The listing builds one solid part. Answer for the finished solid, in the listing's coordinates (mm). A direction names the side the tool comes from. Give positions to 0.01 mm unless a question says otherwise; leave off trailing zeros. Use CSV: the item, a comma, the result in double quotes.
```python
from build123d import *

# Parameters (mm, degrees)
F0_W      = 30
F0_H      = 30
F1_DEPTH  = 15
F3_ANGLE  = 270
F4_R      = 2
F5_R      = 1
F6_DEPTH  = 2
F7_R      = 1
F8_DEPTH  = 2
F10_DEPTH = 2
F11_R     = 1
F12_DEPTH = 2
F13_R     = 1
F14_DEPTH = 2
F15_R     = 1
F16_DEPTH = 2


with BuildPart() as f1:
    # F0 (on Front) → F1 (new body, symmetric)
    with BuildSketch(Plane.XZ):
        Rectangle(F0_W, F0_H)
    extrude(amount=F1_DEPTH, both=True)


with BuildPart() as f1_1:
    # F3: moved
    add(f1.part.rotate(Axis((0, 0.380553, 0), (0, 1, 0)), F3_ANGLE))

    # F4
    f4_edges = [f1_1.edges().sort_by_distance(p)[0] for p in [
        (-15, 0, 15),
        (-15, -15, 0),
        (0, -15, 15),
        (15, -15, 0),
        (15, 0, 15),
        (0, 15, 15),
        (15, 0, -15),
        (0, -15, -15),
        (-15, 0, -15),
        (-15, 15, 0),
        (0, 15, -15),
        (15, 15, 0),
    ]]
    fillet(f4_edges, radius=F4_R)

    # F5 (on face) → F6 (cut)
    with BuildSketch(Plane.XZ.offset(15)):
        Circle(F5_R)
    extrude(amount=-F6_DEPTH, mode=Mode.SUBTRACT)

    # F7 (on face) → F8 (cut)
    with BuildSketch(Plane(origin=(-15, 0, 0), x_dir=(0, -1, 0), z_dir=(-1, 0, 0))):
        with Locations((-10, -10)):
            Circle(F7_R)
        with Locations((10, -10)):
            Circle(F7_R)
        with Locations((10, 10)):
            Circle(F7_R)
        with Locations((-10, 10)):
            Circle(F7_R)
    extrude(amount=-F8_DEPTH, mode=Mode.SUBTRACT)

    # F9 (on face) → F10 (cut)
    with BuildSketch(Plane(origin=(0, 15, 0), x_dir=(-1, 0, 0), z_dir=(0, 1, 0))):
        with BuildLine():
            ThreePointArc((-10, 9), (-9.292893, 9.292893), (-9, 10))
            ThreePointArc((-9, 10), (-10.707107, 10.707107), (-10, 9))
        make_face()
        with BuildLine():
            ThreePointArc((-9, -10), (-9.292893, -9.292893), (-10, -9))
            ThreePointArc((-10, -9), (-10.707107, -10.707107), (-9, -10))
        make_face()
        with BuildLine():
            ThreePointArc((-9, 0), (-9.292893, 0.707107), (-10, 1))
            Line((-10, 1), (-10, -1))
            ThreePointArc((-10, -1), (-9.292893, -0.707107), (-9, 0))
        make_face()
        with BuildLine():
            Line((-10, -1), (-10, 1))
            ThreePointArc((-10, 1), (-11, 0), (-10, -1))
        make_face()
        with BuildLine():
            ThreePointArc((10, -1), (10.707107, -0.707107), (11, 0))
            ThreePointArc((11, 0), (10.707107, 0.707107), (10, 1))
            Line((10, 1), (10, -1))
        make_face()
        with BuildLine():
            ThreePointArc((11, -10), (10.707107, -9.292893), (10, -9))
            ThreePointArc((10, -9), (9.292893, -10.707107), (11, -10))
        make_face()
        with BuildLine():
            ThreePointArc((11, 10), (9.292893, 10.707107), (10, 9))
            ThreePointArc((10, 9), (10.707107, 9.292893), (11, 10))
        make_face()
        with BuildLine():
            Line((10, -1), (10, 1))
            ThreePointArc((10, 1), (9, 0), (10, -1))
        make_face()
    extrude(amount=-F10_DEPTH, mode=Mode.SUBTRACT)

    # F11 (on face) → F12 (cut)
    with BuildSketch(Plane.YZ.offset(15)):
        with Locations((-10, 10)):
            Circle(F11_R)
        with Locations((10, -10)):
            Circle(F11_R)
        Circle(F11_R)
    extrude(amount=-F12_DEPTH, mode=Mode.SUBTRACT)

    # F13 (on face) → F14 (cut)
    with BuildSketch(Plane.XY.offset(15)):
        with Locations((-10, -10)):
            Circle(F13_R)
        with Locations((10, 10)):
            Circle(F13_R)
    extrude(amount=-F14_DEPTH, mode=Mode.SUBTRACT)

    # F15 (on face) → F16 (cut)
    with BuildSketch(Plane(origin=(0, 0, -15), x_dir=(1, 0, 0), z_dir=(0, 0, -1))):
        with Locations((-10, 10)):
            Circle(F15_R)
        with Locations((10, 10)):
            Circle(F15_R)
        with Locations((10, -10)):
            Circle(F15_R)
        with Locations((-10, -10)):
            Circle(F15_R)
        Circle(F15_R)
    extrude(amount=-F16_DEPTH, mode=Mode.SUBTRACT)


solid = f1_1.part
```
Item 1: Which of the six approach directions +Z, -Z, +X, -X, +Y, -Y give full straight-line access (tool end or side, diameter ignored) to faces 4 (the face through (-10, 13, 10)), 5 (the face through (10, 10, -13)), 6 (the face through (13, -10, 10)), 7 (the face through (-14, 10, -9))?
Taken from the geometry:
face 4,"+Y"
face 5,"-Z"
face 6,"+X"
face 7,"-X"
Item 2: Each of these flat-tipped pins is pushed along its axis until it touches: pin 1 (0.6 mm diameter, centred on x = -9.5, z = -10, fed in from +Y); pin 2 (1.8 mm diameter, centred on x = 10, y = 10, fed in from -Z); pin 3 (1.6 mm diameter, centred on y = 10, z = -10, fed in from +X). Where does it stop, or does it pass through?
Taken from the geometry:
pin 1,"y = 13"
pin 2,"z = -13"
pin 3,"x = 13"
Item 3: The mould has two halves that part along Y. Classify faces 1 (the face through (0, 0, 15)), 2 (the face through (14.4, 14.43, 0.18)), 3 (the face through (-10, -10, -13)): +Y half, -Y half, draft (parallel to the pull), parting line (faces both ways), or undercut.
Taken from the geometry:
face 1,"draft"
face 2,"+Y half"
face 3,"undercut"
Item 4: Find the intervals of material crossed by line 1 along X through (y, z) = (13.45, 10); line 2 along X through (y, z) = (-10, -13.9); line 3 along Z through (x, y) = (-13.5, -10), in increasing order.
Taken from the geometry:
line 1,"-14.95 to -11, -9 to 9, 11 to 14.95"
line 2,"-14.79 to -11, -9 to 9, 11 to 14.79"
line 3,"-14.94 to -11, -9 to 9, 11 to 14.94"
